Design review of the part built by this model. Coordinates are the model's own, in mm. Face numbers are marked on the shaded views. A direction names the side the tool comes from. Coordinates: 2 decimals unless noted, no trailing zeros. Loops run counter-clockwise (first coordinate to the right, second up) from the corner with the lowest first, then second, coordinate; pieces in that order, holes last.
Q1. Draft analysis for pull direction Y (two halves, no side actions). For the marked faces 6, 7 and 8, state which applies: released by +Y, released by -Y, zero draft, split by the parting line, or undercut.
Q2. Add section C-C on y = 11.5. Give the boundary of the cut face in (x, z) (3 decimals).
Q3. Add section B-B on y = 39. Give the boundary of the cut face in (x, z), and give its area (3 significant figures).
Q4. Wall thickness on probe 1 along Y at (x, z) = (0, -8.75) (3 decimals); probe 2 along Z at (x, y) = (0, 9.75) (3 decimals); probe 3 along X at (y, z) = (16.5, -9) (3 decimals): over which ranges is each line inside the solid? List them lowest first.
Q5. Add section D-D on x = 7. Give the boundary of the cut face in (y, z), and give its area (3 significant figures).
Q6. Machinability: for the marked faces 1, 2, 3, 4 and 5, which of the approach directions +Z, -Z, +X, -X, +Y, -Y give a long, thin tool a straight path to every point of the face, cutting with its end or side? Answer none if there is none.
Q7. For P1, Ø5.5, axis at x = 3, z = -7, coming from the -Y side; P2, Ø4.5, axis at x = 0, y = 55.5, coming from the +Z side (3 decimals); P3, Ø2.5, axis at x = 0, y = 55.5, coming from the -Z side, all flat-tipped, find the tip position at first contact; note any pin that passes through.
Q8. Add section A-A on z = 8. Give the boundary of the cut face in (x, y), and give its area (3 significant figures).
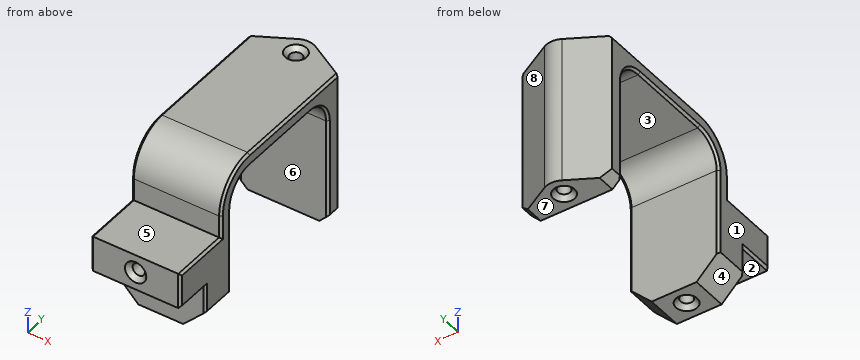
```python
from build123d import *

# Parameters (mm, degrees)
BOX_W             = 10
BOX_H             = 50
BOX_DEPTH         = 33
SKETCH005_W       = 31
SKETCH005_H       = 30
SKETCH005_W_2     = 13
SKETCH005_H_2     = 14
SKETCH005_W_3     = 8
SKETCH005_H_3     = 11
POCKET003_DEPTH   = 10
CHAMFER009_SIZE   = 5
FILLET004_1_R     = 9
FILLET004_2_R     = 6
SKETCH010_R       = 1.375
POCKET006_DEPTH   = 8
SKETCH011_R       = 1.375
POCKET007_DEPTH   = 8
CHAMFER011_SIZE   = 1
PAD004_DEPTH      = 33
SKETCH016_R       = 1.375
POCKET011_DEPTH   = 8
SKETCH025_R       = 1.375
POCKET017_DEPTH   = 8
CHAMFER012_1_SIZE = 2
CHAMFER012_2_SIZE = 1
CHAMFER015_SIZE   = 0.5


with BuildPart() as batterybracketbatteryfillet004:
    # Box → Box (new body)
    with BuildSketch(Plane(origin=(0, 4.5, -15), x_dir=(1, 0, 0), z_dir=(0, 0, 1))):
        with Locations((5, 25)):
            Rectangle(BOX_W, BOX_H)
    extrude(amount=BOX_DEPTH)

    # Sketch005 → Pocket003 (cut)
    with BuildSketch(Plane(origin=(10, 4.5, -15), x_dir=(0, 1, 0), z_dir=(1, 0, 0))):
        with Locations((31.5, 15)):
            Rectangle(SKETCH005_W, SKETCH005_H)
        with Locations((6.5, 26)):
            Rectangle(SKETCH005_W_2, SKETCH005_H_2)
        with Locations((4, 5.5)):
            Rectangle(SKETCH005_W_3, SKETCH005_H_3)
    extrude(amount=-POCKET003_DEPTH, mode=Mode.SUBTRACT)

    # Chamfer009
    chamfer009_edges = [batterybracketbatteryfillet004.edges().sort_by_distance(p)[0] for p in [
        (10, 16.5, -15),
    ]]
    chamfer(chamfer009_edges, length=CHAMFER009_SIZE)

    # Fillet004 1
    fillet004_1_edges = [batterybracketbatteryfillet004.edges().sort_by_distance(p)[0] for p in [
        (5, 17.5, 18),
    ]]
    fillet(fillet004_1_edges, radius=FILLET004_1_R)

    # Fillet004 2
    fillet004_2_edges = [batterybracketbatteryfillet004.edges().sort_by_distance(p)[0] for p in [
        (5, 20.5, 15),
        (5, 51.5, 15),
    ]]
    fillet(fillet004_2_edges, radius=FILLET004_2_R)


with BuildPart() as batterybracketprintingchamfer021_final:
    # Part__Mirroring003: instance of BatteryBracketBatteryFillet004
    add(batterybracketbatteryfillet004.part.mirror(Plane(origin=(0, 0, 0), x_dir=(0, -1, 0), z_dir=(1, 0, 0))))

    # Fusion: union BatteryBracketBatteryFillet004
    add(batterybracketbatteryfillet004.part)

    # Sketch010 → Pocket006 (cut)
    with BuildSketch(Plane.XZ.offset(-4.5)):
        Circle(SKETCH010_R)
    extrude(amount=-POCKET006_DEPTH, mode=Mode.SUBTRACT)

    # Sketch011 → Pocket007 (cut)
    with BuildSketch(Plane(origin=(0, 0, -15), x_dir=(1, 0, 0), z_dir=(0, 0, -1))):
        with Locations((0, -16.5)):
            Circle(SKETCH011_R)
    extrude(amount=-POCKET007_DEPTH, mode=Mode.SUBTRACT)

    # Chamfer011
    chamfer011_edges = [batterybracketprintingchamfer021_final.edges().sort_by_distance(p)[0] for p in [
        (-1.375, 4.5, 0),
        (-1.375, 16.5, -15),
    ]]
    chamfer(chamfer011_edges, length=CHAMFER011_SIZE)

    # Sketch015 → Pad004 (new body)
    with BuildSketch(Plane.XY.offset(18)):
        with BuildLine():
            Line((10, 54.5), (1.949289, 58.992889))
            ThreePointArc((1.949289, 58.992889), (0, 59.5), (-1.949289, 58.992889))
            Line((-1.949289, 58.992889), (-10, 54.5))
            Line((-10, 54.5), (10, 54.5))
        make_face()
    extrude(amount=-PAD004_DEPTH)

    # Sketch016 → Pocket011 (cut)
    with BuildSketch(Plane.XY.offset(18)):
        with Locations((0, 55.5)):
            Circle(SKETCH016_R)
    extrude(amount=-POCKET011_DEPTH, mode=Mode.SUBTRACT)

    # Sketch025 → Pocket017 (cut)
    with BuildSketch(Plane(origin=(0, 0, -15), x_dir=(1, 0, 0), z_dir=(0, 0, -1))):
        with Locations((0, -55.5)):
            Circle(SKETCH025_R)
    extrude(amount=-POCKET017_DEPTH, mode=Mode.SUBTRACT)

    # Chamfer012 1
    chamfer012_1_edges = [batterybracketprintingchamfer021_final.edges().sort_by_distance(p)[0] for p in [
        (-10, 53, -15),
        (10, 53, -15),
    ]]
    chamfer(chamfer012_1_edges, length=CHAMFER012_1_SIZE)

    # Chamfer012 2
    chamfer012_2_edges = [batterybracketprintingchamfer021_final.edges().sort_by_distance(p)[0] for p in [
        (-1.375, 55.5, -15),
        (-1.375, 55.5, 18),
    ]]
    chamfer(chamfer012_2_edges, length=CHAMFER012_2_SIZE)

    # Chamfer015
    chamfer015_edges = [batterybracketprintingchamfer021_final.edges().sort_by_distance(p)[0] for p in [
        (-10, 51.5, -2),
        (-10, 49.742641, 13.242641),
        (-10, 36, 15),
        (-10, 40.5, 18),
        (-10, 22.257359, 13.242641),
        (-10, 20.136039, 15.363961),
        (-10, 20.5, -0.5),
        (-10, 17.5, 6.5),
        (-10, 11, 4),
        (-10, 12.5, -7),
        (-10, 4.5, 0),
        (-10, 8.5, -4),
        (10, 51.5, -2),
        (10, 36, 15),
        (10, 40.5, 18),
        (10, 20.5, -0.5),
        (10, 17.5, 6.5),
        (10, 11, 4),
        (10, 12.5, -7),
        (10, 4.5, 0),
        (10, 8.5, -4),
        (10, 49.742641, 13.242641),
        (10, 22.257359, 13.242641),
        (10, 20.136039, 15.363961),
    ]]
    chamfer(chamfer015_edges, length=CHAMFER015_SIZE)


solid = batterybracketprintingchamfer021_final.part
```
Entries:
1. face 6: undercut
1. face 7: zero draft
1. face 8: released by +Y
2. outline: (-10, -3.5) - (-9.5, -4) - (9.5, -4) - (10, -3.5) - (10, 3.5) - (9.5, 4) - (-9.5, 4) - (-10, 3.5) - close; hole circle Ø2.75 at (0, 0)
3. outline: (-10, 15.5) - (-9.5, 15) - (9.5, 15) - (10, 15.5) - (10, 17.5) - (9.5, 18) - (-9.5, 18) - (-10, 17.5) - close
3. area: 59.5 mm2
4. probe 1: y = 12.5 to 15.125, 17.875 to 20.5, 51.5 to 54.125, 56.875 to 59.5
4. probe 2: z = -4 to -1.375, 1.375 to 4
4. probe 3: x = -10 to -1.375, 1.375 to 10
5. outline: (4.5, -4) - (12.5, -4) - (12.5, -13) - (20.5, -13) - (20.5, 9) arc R6 cw to (26.5, 15) - (45.5, 15) arc R6 cw to (51.5, 9) - (51.5, -15) - (56.17, -15) - (56.17, 18) - (26.5, 18) arc R9 ccw to (17.5, 9) - (17.5, 4) - (4.5, 4) - close
5. area: 487 mm2
6. face 1: +Z, -Z, -X, +Y, -Y
6. face 2: -Z, +X, -X, -Y
6. face 3: -Z, +X, -X
6. face 4: -Z, -X, -Y
6. face 5: +Z, +X, -X, -Y
7. P1: stops at y = 12.5
7. P2: stops at z = 17.875
7. P3: stops at z = -7
8. outline: (-10, 18) - (-9.5, 17.5) - (9.5, 17.5) - (10, 18) - (10, 20) - (9.5, 20.5) - (-9.5, 20.5) - (-10, 20) - close; (-10, 52) - (-9.5, 51.5) - (9.5, 51.5) - (10, 52) - (10, 54.5) - (1.95, 58.99) arc R4 ccw to (-1.95, 58.99) - (-10, 54.5) - close
8. area: 174 mm2
